The listing builds one solid part. Answer for the finished solid, in the listing's coordinates (mm). A direction names the side the tool comes from. Coordinates: 2 decimals unless noted, no trailing zeros. Order: outer loops, then holes, each group sorted by start corner. A loop starts at its lowest first (then second) coordinate and runs counter-clockwise, first axis right, second up. Notation, with made-up numbers: (-18.5, 77) - (1.5, 77) arc R26 cw to (1.5, 92) - close; hole circle Ø3 at (15.25, -35). An arc over 180 degrees is marked (long way). One line per item, written item: value. Start each with the question number.
```python
from build123d import *

# Parameters (mm, degrees)
F0_R     = 104
F1_DEPTH = 25
F2_R     = 75
F3_DEPTH = 15
F4_R     = 3
F5_SIZE  = 2
F7_D     = 14


with BuildPart() as f1:
    # F0 (on Right) → F1 (new body)
    with BuildSketch(Plane.YZ):
        Circle(F0_R)
    extrude(amount=-F1_DEPTH)

    # F2 (on face) → F3 (cut)
    with BuildSketch(Plane(origin=(-25, 0, 0), x_dir=(0, -1, 0), z_dir=(-1, 0, 0))):
        Circle(F2_R)
    extrude(amount=-F3_DEPTH, mode=Mode.SUBTRACT)

    # F4
    f4_edges = [f1.edges().sort_by_distance(p)[0] for p in [
        (-10, 75, 0),
    ]]
    fillet(f4_edges, radius=F4_R)

    # F5
    f5_edges = [f1.edges().sort_by_distance(p)[0] for p in [
        (0, -104, 0),
    ]]
    chamfer(f5_edges, length=F5_SIZE)

    # F7 (through all)
    with Locations(Plane.YZ):
        with Locations((0, 93), (93, 0), (0, -93), (-93, 0)):
            Hole(F7_D / 2)


solid = f1.part
```
(1) The part is cut by section C-C on x = -18.25. Determine the outline of the cut face in (y, z).
(2) Flat-ended cylindrical pins translate along their axes: pin 1 Ø4 at (x, z) = (-11.5, 36.5) entering from -Y; pin 2 Ø4 at (x, z) = (-16.5, -39.5) entering from -Y; pin 3 Ø6 at (x, z) = (-15.5, -56) entering from -Y. Find the tip coordinate at first contact, or state that the pin passes through.
(3) Consider probe 1 along Z at (x, y) = (-16.25, 0); probe 2 along X at (y, z) = (-10.5, 30); probe 3 along Y at (x, z) = (-19.75, 16.5). Determine where each line is inside the solid, lowest interval first.
(4) For a pull along Y with two mould halves and no side action, classify faces 1 (the face through (-13, -86, 0)), 2 (the face through (-13.339, -82.531, -63.282)), 3 (the face through (0, -1, 1)) as pulls with the +Y half, pulls with the -Y half, needs draft (parallel to the pull), parting line crosses it, or undercut.
(5) The part is cut by section A-A on y = 0. Determine the outline of the cut face in (x, z), plus the area to 3 significant figures.
(6) For faces 4 (the face through (-10, 1, 1)), 5 (the face through (-12.68, 0.91, 99.94)), determine the directions among +Z, -Z, +X, -X, +Y, -Y from which every point of the face is accessible in a straight line to the end or side of a thin tool.
Completed:
1. outline: circle Ø208 at (0, 0); hole circle Ø14 at (-93, 0); hole circle Ø150 at (0, 0); hole circle Ø14 at (0, -93); hole circle Ø14 at (0, 93); hole circle Ø14 at (93, 0)
2. pin 1: stops at y = -98.11
2. pin 2: stops at y = -97
2. pin 3: stops at y = -89.48
3. probe 1: z = -104 to -100, -86 to -75, 75 to 86, 100 to 104
3. probe 2: x = -10 to 0
3. probe 3: y = -102.68 to -73.16, 73.16 to 102.68
4. face 1: undercut
4. face 2: parting line crosses it
4. face 3: needs draft
5. outline: (-25, -104) - (-2, -104) - (0, -102) - (0, -100) - (-25, -100) - close; (-25, -86) - (0, -86) - (0, 86) - (-25, 86) - (-25, 75) - (-13, 75) arc R3 cw to (-10, 72) - (-10, -72) arc R3 cw to (-13, -75) - (-25, -75) - close; (-25, 100) - (0, 100) - (0, 102) - (-2, 104) - (-25, 104) - close
5. area: 2,250 mm2
6. face 4: -X
6. face 5: +X, -X
